Geometry check sheet. Reference: the model listing, model coordinates, mm. Face numbers are marked on the shaded views. A direction names the side the tool comes from. Give positions to 0.01 mm unless a question says otherwise; leave off trailing zeros. Write each loop counter-clockwise with the first axis right and the second up, starting at its lowest first coordinate (ties: lowest second). Pieces come first, ordered by that corner, then holes. Notation, with made-up numbers: M 43.25,-3 L 95.25,-3 A24 cw 95.25,19 Z; hole C 69.5,-18.75 d2. An arc over 180 degrees is marked long. Write each question's results on one line, items separated by ' | '.
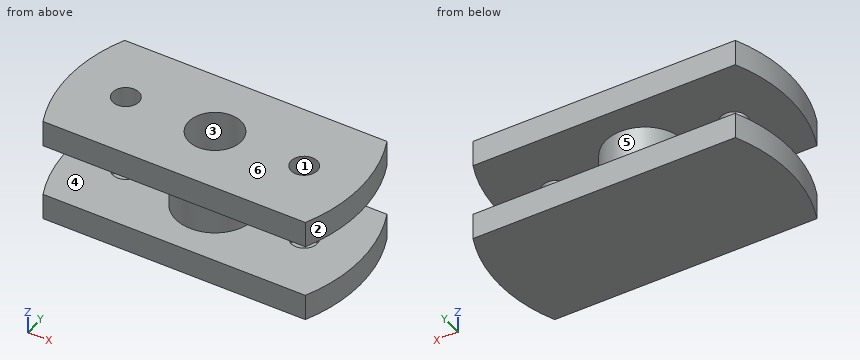
```python
from build123d import *

# Parameters (mm, degrees)
BOSS_EXTRUDE1_DEPTH = 5
SKETCH2_R           = 7.5
BOSS_EXTRUDE2_DEPTH = 10
SKETCH3_R           = 2.5
CUT_EXTRUDE1_DEPTH  = 2
SKETCH4_R           = 7.5
BOSS_EXTRUDE3_DEPTH = 5
SKETCH6_R           = 7.5
BOSS_EXTRUDE4_DEPTH = 5
SKETCH7_R           = 5
CUT_EXTRUDE2_DEPTH  = 15
SKETCH8_R           = 2.5
CUT_EXTRUDE3_DEPTH  = 5


with BuildPart() as part:
    # Sketch1 → Boss-Extrude1 (new body)
    with BuildSketch(Plane.XY):
        with BuildLine():
            Line((-25, -12.5), (25, -12.5))
            ThreePointArc((25, -12.5), (27.728219713, 0), (25, 12.5))
            Line((25, 12.5), (-25, 12.5))
            ThreePointArc((-25, 12.5), (-27.728219713, 0), (-25, -12.5))
        make_face()
    extrude(amount=BOSS_EXTRUDE1_DEPTH)

    # Sketch2 → Boss-Extrude2 (add)
    with BuildSketch(Plane.XY.offset(5)):
        Circle(SKETCH2_R)
    extrude(amount=BOSS_EXTRUDE2_DEPTH)

    # Sketch3 → Cut-Extrude1 (cut)
    with BuildSketch(Plane.XY.offset(5)):
        with Locations((17, 0)):
            Circle(SKETCH3_R)
        with Locations((-17, 0)):
            Circle(SKETCH3_R)
    extrude(amount=-CUT_EXTRUDE1_DEPTH, mode=Mode.SUBTRACT)



with BuildPart() as body_2:
    # Sketch4 → Boss-Extrude3 (new body)
    with BuildSketch(Plane.XY.offset(15)):
        with BuildLine():
            Line((25, 12.5), (-25, 12.5))
            ThreePointArc((-25, 12.5), (-27.728219713, 0), (-25, -12.5))
            Line((-25, -12.5), (25, -12.5))
            ThreePointArc((25, -12.5), (27.728219713, 0), (25, 12.5))
        make_face()
        Circle(SKETCH4_R, mode=Mode.SUBTRACT)
    extrude(amount=BOSS_EXTRUDE3_DEPTH)


with BuildPart() as part_1:
    add(part.part)

    add(body_2.part)  # Boss-Extrude4 merges body 2
    # Sketch6 → Boss-Extrude4 (add)
    with BuildSketch(Plane.XY.offset(15)):
        Circle(SKETCH6_R)
    extrude(amount=BOSS_EXTRUDE4_DEPTH)

    # Sketch7 → Cut-Extrude2 (cut)
    with BuildSketch(Plane.XY.offset(20)):
        Circle(SKETCH7_R)
    extrude(amount=-CUT_EXTRUDE2_DEPTH, mode=Mode.SUBTRACT)

    # Sketch8 → Cut-Extrude3 (cut)
    with BuildSketch(Plane.XY.offset(20)):
        with Locations((17, 0)):
            Circle(SKETCH8_R)
        with Locations((-17, 0)):
            Circle(SKETCH8_R)
    extrude(amount=-CUT_EXTRUDE3_DEPTH, mode=Mode.SUBTRACT)


solid = part_1.part
```
Q1. Release check for a two-part mould opening along Z. For the marked faces 3, 4, 5 and 6 record: released by +Z, released by -Z, zero draft, split by the parting line, or undercut.
Answer key:
face 3: zero draft | face 4: undercut | face 5: undercut | face 6: released by +Z
Q2. Section check D-D (x = 17). Enter the section's corners in (y, z), then the cut area to 3 significant figures.
Answer key:
outline: M -12.5,0 L 12.5,0 L 12.5,5 L 2.5,5 L 2.5,3 L -2.5,3 L -2.5,5 L -12.5,5 Z; M -12.5,15 L -2.5,15 L -2.5,20 L -12.5,20 Z; M 2.5,15 L 12.5,15 L 12.5,20 L 2.5,20 Z | area: 215 mm2
Q3. Section check B-B (x = -20.5). Enter the section's corners in (y, z), then the cut area to 3 significant figures.
Answer key:
outline: M -12.5,0 L 12.5,0 L 12.5,5 L -12.5,5 Z; M -12.5,15 L 12.5,15 L 12.5,20 L -12.5,20 Z | area: 250 mm2
Q4. Material ranges on probe 1 along Z at (x, y) = (-7.5, -9.5); probe 2 along Y at (x, z) = (0, 10); probe 3 along Y at (x, z) = (-17, 4), recorded low to high. Write a range as [from, to].
Answer key:
probe 1: z = [0, 5], [15, 20] | probe 2: y = [-7.5, -5], [5, 7.5] | probe 3: y = [-12.5, -2.5], [2.5, 12.5]
Q5. Section check A-A (y = 0). State how many separate pieces and enclosed holes the cut face has, then the cut area to 3 significant figures.
Answer key:
separate pieces: 3 | enclosed holes: 0 | area: 485 mm2
Q6. Access from +Z, -Z, +X, -X, +Y, -Y to the whole of each face (thin tool, end or side, straight path). Record for the marked faces 1 and 2.
Answer key:
face 1: +Z | face 2: +Z, -Z, +X
Q7. Depth check by flat-ended pin: P1, Ø2.5, axis at x = -16.5, y = -0.5, coming from the +Z side; P2, Ø5, axis at y = -2.5, z = 8.5, coming from the +X side; P3, Ø8, axis at x = 9.5, z = 10.5, coming from the -Y side. Enter the tip coordinate at first touch or a pass-through.
Answer key:
P1: stops at z = 3 | P2: stops at x = 7.5 | P3: stops at y = -5.1
Q8. Section check C-C (z = 16.25). Enter the section's corners in (x, y), then the cut area to 3 significant figures.
Answer key:
outline: M -25,-12.5 L 25,-12.5 A30 ccw 25,12.5 L -25,12.5 A30 ccw Z; hole C -17,0 d5; hole C 0,0 d10; hole C 17,0 d5 | area: 1,220 mm2
